Print and shaded views of the part. All mm, measured from the part's lowest x, y and z. A direction names the side the tool comes from. Give positions to 0.01 mm unless a question says otherwise; leave off trailing zeros. Write each loop counter-clockwise with the first axis right and the second up, starting at its lowest first coordinate (ties: lowest second). Pieces come first, ordered by that corner, then holes. Notation, with made-up numbers: M 77,49.25 L 110,49.25 A12 cw 110,71.25 Z; hole C 8.25,-32 d5. An arc over 180 degrees is marked long. One line per question, with ' | ' between items. Start each with the question number.
1. Cut at D-D, the plane x = 3. Write the cut outline in (y, z), then the cut area to 3 significant figures.
2. Which spindle directions (+Z, -Z, +X, -X, +Y, -Y) get a long thin tool onto all of the face, cutting with end or side? Do the marked faces 1, 2 and 3. Say none if no direction does.
3. Flat gauge pins, fed straight in: pin 1 (0.9 mm diameter, centred on y = 2, z = 1.5, fed in from -X); pin 2 (1.1 mm diameter, centred on x = 18, z = 1.5, fed in from -Y); pin 3 (2 mm diameter, centred on x = 4, y = 7.5, fed in from +Z). Where does each tip first touch, or does it go through?
4. Cut at C-C, the plane y = 10.1. Write the cut outline in (x, z).
5. Cut at B-B, the plane z = 0.3. Write the cut outline in (x, y).
6. Cut at A-A, the plane x = 6. Write the cut outline in (y, z).
7. Wall check: L1, parallel to Y at x = 20, z = 1.6; L2, parallel to Y at x = 6, z = 1.35; L3, parallel to X at y = 1, z = 1.8. Give the ranges that are in metal, low to high.
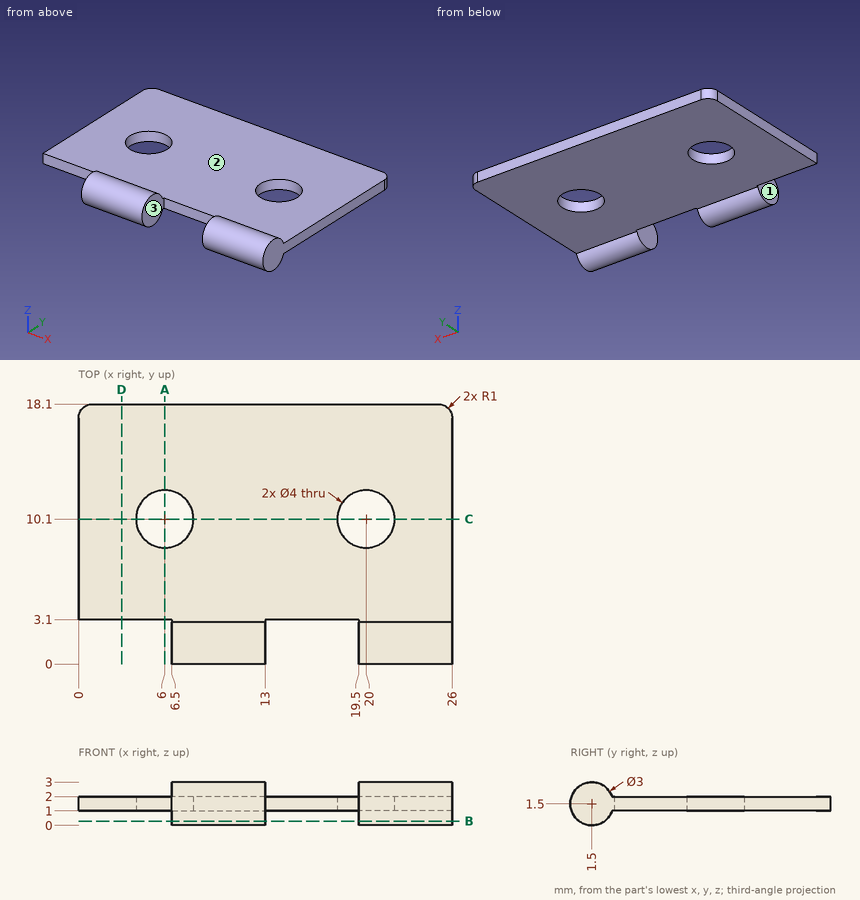
Here are the results:
1) outline: M 3.1,1 L 18.1,1 L 18.1,2 L 3.1,2 Z | area: 15.0 mm^2
2) face 1: +Z, -Z, -X, -Y | face 2: +Z, +X, -X, +Y | face 3: +Z, -Z, -Y
3) pin 1: x = 6.5 | pin 2: y = 3.1 | pin 3: z = 2
4) outline: M 0,1 L 4,1 L 4,2 L 0,2 Z; M 8,1 L 18,1 L 18,2 L 8,2 Z; M 22,1 L 26,1 L 26,2 L 22,2 Z
5) outline: M 6.5,0.6 L 13,0.6 L 13,2.4 L 6.5,2.4 Z; M 19.5,0.6 L 26,0.6 L 26,2.4 L 19.5,2.4 Z
6) outline: M 3.1,1 L 8.1,1 L 8.1,2 L 3.1,2 Z; M 12.1,1 L 18.1,1 L 18.1,2 L 12.1,2 Z
7) L1: 0 to 8.1, 12.1 to 18.1 | L2: 3.1 to 8.1, 12.1 to 18.1 | L3: 6.5 to 13, 19.5 to 26
